```python
from build123d import *

# Parameters (mm, degrees)
SKETCH1_W                      = 31.75
SKETCH1_H                      = 152.4
BOSS_EXTRUDE1_DEPTH            = 4.7625
M3X0_5_TAPPED_HOLE1_AT_2_COUNT = 2
M3X0_5_TAPPED_HOLE1_AT_2_PITCH = 19.05
F_12_0MM_DOWEL_HOLE1_D         = 12
CUT_EXTRUDE1_DEPTH             = 79.416715374


with BuildPart() as part:
    # Sketch1 → Boss-Extrude1 (new, symmetric)
    with BuildSketch(Plane(origin=(0, 0, 0), x_dir=(0, 0, -1), z_dir=(1, 0, 0))):
        Rectangle(SKETCH1_W, SKETCH1_H)
    extrude(amount=BOSS_EXTRUDE1_DEPTH, both=True)

    # Sketch4 → M3x0.5 Tapped Hole1 (revolve, cut)
    with BuildSketch(Plane(origin=(0, 76.2, -9.525), x_dir=(0, 0, 1), z_dir=(1, 0, 0))):
        Polygon((0, 0), (0, 13.451075774), (1.25, 12.7), (1.25, 0), align=None)
    m3x0_5_tapped_hole1 = revolve(axis=Axis((0, 82.55, -9.525), (0, -1, 0)), mode=Mode.SUBTRACT)

    # M3x0.5 Tapped Hole1 at 2: M3x0.5 Tapped Hole1 ×2
    with Locations(*[(0, 0, i * M3X0_5_TAPPED_HOLE1_AT_2_PITCH) for i in range(1, M3X0_5_TAPPED_HOLE1_AT_2_COUNT)]):
        add(m3x0_5_tapped_hole1, mode=Mode.SUBTRACT)

    # Mirror1: M3x0.5 Tapped Hole1 across plane
    add(m3x0_5_tapped_hole1.mirror(Plane.ZX), mode=Mode.SUBTRACT)

    # Mirror1 copy 1 sketch → Mirror1 copy 1 (revolve, cut)
    with BuildSketch(Plane(origin=(0, -76.2, 9.525), x_dir=(0, 0, 1), z_dir=(1, 0, 0))):
        Polygon((0, 0), (0, -13.451075774), (1.25, -12.7), (1.25, 0), align=None)
    revolve(axis=Axis((0, -82.55, 9.525), (0, -1, 0)), mode=Mode.SUBTRACT)

    # Ø12.0mm Dowel Hole1 (through all)
    with Locations(Plane(origin=(4.7625, 0, 0), x_dir=(0, 0, -1), z_dir=(1, 0, 0))):
        with Locations((0, 0)):
            Hole(F_12_0MM_DOWEL_HOLE1_D / 2)

    # Sketch9 → Cut-Extrude1 (cut, through all)
    with BuildSketch(Plane(origin=(4.7625, 0, 0), x_dir=(0, 0, -1), z_dir=(1, 0, 0))):
        with BuildLine():
            Line((9.525, 50.8), (9.525, 25.4))
            ThreePointArc((9.525, 25.4), (0, 15.875), (-9.525, 25.4))
            Line((-9.525, 25.4), (-9.525, 50.8))
            ThreePointArc((-9.525, 50.8), (0, 60.325), (9.525, 50.8))
        make_face()
        with BuildLine():
            Line((9.525, -25.4), (9.525, -50.8))
            ThreePointArc((9.525, -50.8), (0, -60.325), (-9.525, -50.8))
            Line((-9.525, -50.8), (-9.525, -25.4))
            ThreePointArc((-9.525, -25.4), (0, -15.875), (9.525, -25.4))
        make_face()
    extrude(amount=-CUT_EXTRUDE1_DEPTH, mode=Mode.SUBTRACT)


solid = part.part
```
Geometry check sheet. Reference: the model listing, model coordinates, mm. A direction names the side the tool comes from. Coordinates: 2 decimals unless noted, no trailing zeros. Order: outer loops, then holes, each group sorted by start corner. A loop starts at its lowest first (then second) coordinate and runs counter-clockwise, first axis right, second up. Notation, with made-up numbers: (9, 35.25) - (58, 35.25) arc R32 ccw to (58, 62.25) - close; hole circle Ø10 at (-31, 78). An arc over 180 degrees is marked (long way). Answer as a JSON object with one key per item and string values. Group by question number.
Item 1: Sectioned sample at A-A, the plane y = 0. Record the cut outline in (x, z) (1 decimal), and give its area (3 significant figures).
Item 2: Scan lines: probe 1 along Z at (x, y) = (0, -68.25) (3 decimals); probe 2 along Y at (x, z) = (-4, 0) (3 decimals); probe 3 along Y at (x, z) = (-2.5, 7). Record each from-to range of solid material in increasing order.
Item 3: Sectioned sample at D-D, the plane y = 49. Record the cut outline in (x, z) (1 decimal), and give its area (3 significant figures).
Item 4: Depth check by flat-ended pin: pin 1 Ø1.5 at (x, z) = (0, -9.525) entering from -Y; pin 2 Ø11 at (y, z) = (0, 0) entering from -X; pin 3 Ø3 at (x, z) = (0, 9.525) entering from -Y. Enter the tip coordinate at first touch or a pass-through.
Item 5: Sectioned sample at B-B, the plane x = -3. Record the cut outline in (y, z) (3 decimals), and give its area (3 significant figures).
Item 6: Tool access check on faces 1 (the face through (1.22, -69.94, -9.8)), 2 (the face through (1.22, 69.94, -9.8)), 3 (the face through (0.067, 15.877, -0.209)). Record the directions out of +Z, -Z, +X, -X, +Y, -Y that give a thin tool (end or side, any length) a straight path to the whole face; none if there is none.
Item 7: Draft check along Z on faces 4 (the face through (0, 38, 9.525)), 5 (the face through (4.762, 1, -7)), 6 (the face through (0, -1, 15.875)), 7 (the face through (0, -38, -9.525)). Enter one of: +Z half, -Z half, draft (parallel to the pull), parting line (faces both ways), or undercut.
Item 8: Sectioned sample at C-C, the plane z = 2.5. Record the cut outline in (x, y), and give its area (3 significant figures).
Resolved:
{
 "1": {"outline": "(-4.8, -15.9) - (4.8, -15.9) - (4.8, -6) - (-4.8, -6) - close; (-4.8, 6) - (4.8, 6) - (4.8, 15.9) - (-4.8, 15.9) - close", "area": "188 mm^2"},
 "2": {"probe 1": "-15.875 to -10.775, -8.275 to 8.275, 10.775 to 15.875", "probe 2": "-76.2 to -60.325, -15.875 to -6, 6 to 15.875, 60.325 to 76.2", "probe 3": "-76.2 to -57.26, -18.94 to 18.94, 57.26 to 76.2"},
 "3": {"outline": "(-4.8, -15.9) - (4.8, -15.9) - (4.8, -9.5) - (-4.8, -9.5) - close; (-4.8, 9.5) - (4.8, 9.5) - (4.8, 15.9) - (-4.8, 15.9) - close", "area": "121 mm^2"},
 "4": {"pin 1": "y = -63.2", "pin 2": "through", "pin 3": "y = -76.2"},
 "5": {"outline": "(-76.2, -15.875) - (76.2, -15.875) - (76.2, 15.875) - (-76.2, 15.875) - close; hole (-50.8, -9.525) - (-25.4, -9.525) arc R9.525 ccw to (-25.4, 9.525) - (-50.8, 9.525) arc R9.525 ccw to start; hole circle Ø12 at (0, 0); hole (25.4, -9.525) - (50.8, -9.525) arc R9.525 ccw to (50.8, 9.525) - (25.4, 9.525) arc R9.525 ccw to start", "area": "3,190 mm^2"},
 "6": {"face 1": "-Y", "face 2": "+Y", "face 3": "+X, -X"},
 "7": {"face 4": "undercut", "face 5": "draft", "face 6": "+Z half", "face 7": "undercut"},
 "8": {"outline": "(-4.76, -76.2) - (4.76, -76.2) - (4.76, -59.99) - (-4.76, -59.99) - close; (-4.76, -16.21) - (4.76, -16.21) - (4.76, -5.45) - (-4.76, -5.45) - close; (-4.76, 5.45) - (4.76, 5.45) - (4.76, 16.21) - (-4.76, 16.21) - close; (-4.76, 59.99) - (4.76, 59.99) - (4.76, 76.2) - (-4.76, 76.2) - close", "area": "514 mm^2"}
}
